Can you work these out from the model? Positions are in its coordinate system, mm. Face numbers are marked on the shaded views. A direction names the side the tool comes from. Round coordinates to 2 decimals unless told otherwise and drop trailing zeros. Write each loop counter-clockwise with the first axis right and the second up, starting at its lowest first coordinate (ties: lowest second). Pieces come first, ordered by that corner, then holes. Notation, with made-up numbers: M 42.25,-25.5 L 68.25,-25.5 A21 cw 68.25,-14.5 Z; hole C 86.25,-36 d8. An arc over 180 degrees is marked long. Answer in a Markdown table with one row per item. Add a question column.
(1) Suppose I cut it at D-D, the plane x = -4. Write out the boundary of the cut face in (y, z), then the cut area to 3 significant figures.
(2) If I drill on probe 1 along Y at (x, z) = (19, -2.2); probe 2 along X at (y, z) = (-20.5, -8.25); probe 3 along Y at (x, z) = (33, -4.5), over which ranges is the centre line in solid material (lowest first)?
(3) Suppose I cut it at B-B, the plane y = -16.5. Write out the boundary of the cut face in (x, z).
(4) Suppose I cut it at C-C, the plane z = -5.75. Write out the boundary of the cut face in (x, y), then the cut area to 3 significant figures.
(5) Suppose I cut it at A-A, the plane x = -30. Write out the boundary of the cut face in (y, z).
(6) For the marked faces 1 and 2, which set-ups out of +Z, -Z, +X, -X, +Y, -Y let a thin tool reach every point of the face, with its end or its side?
(7) I'm going to push flat-ended pins straight in: pin 1 (5 mm diameter, centred on x = -18.5, z = -3, fed in from +Y); pin 2 (2 mm diameter, centred on x = 19, y = 25, fed in from -Z); pin 3 (2.5 mm diameter, centred on x = -39, y = -24.5, fed in from -Z). Where does each tip first touch, or does it pass through?
(8) If we mould it in two halves opening along X, with no side actions, what happens to the marked faces 3, 4, 5 and 6? For each: released by +X, released by -X, zero draft, split by the parting line, or undercut.
Autodesk Inventor part; units mm, degrees
ref_plane "YZ Plane" through (0, 0, 0) normal (1, 0, 0) x (0, 1, 0)
ref_plane "XZ Plane" through (0, 0, 0) normal (0, 1, 0) x (-1, 0, 0)
ref_plane "XY Plane" through (0, 0, 0) normal (0, 0, 1) x (1, 0, 0)
ref_plane "Work Plane1" through (0, 0, 0) normal (0, 0, 1) x (1, 0, 0)
sketch "Sketch1" plane through (0, 0, 0) normal (0, 0, 1) x (1, 0, 0)
  line L0 (47, 31) -> (-47, 31)
  line L1 (-47, 31) -> (-47, -31)
  line L2 (-47, -31) -> (47, -31)
  line L3 (47, -31) -> (47, 31)
  line L4 (47, 31) -> (-47, -31) construction
  line L5 (-47, 31) -> (47, -31) construction
  point P0 (0, 0)
  dimension "d0" = 94
  dimension "d1" = 62
extrude "Extrusion1" add sketch "Sketch1" along normal blind 2
sketch "Sketch2" plane through (0, 0, 0) normal (0, 0, -1) x (-1, 0, 0)
  circle A0 centre (39, 24.5) radius 3
  circle A1 centre (39, 24.5) radius 1.35
  circle A2 centre (39, -24.5) radius 3
  circle A3 centre (39, -24.5) radius 1.35
  circle A4 centre (-19, -24.5) radius 3
  circle A5 centre (-19, -24.5) radius 1.35
  circle A6 centre (-19, 24.5) radius 3
  circle A7 centre (-19, 24.5) radius 1.35
  point P0 (0, 0)
extrude "Extrusion2" add sketch "Sketch2" along normal blind 3
sketch "Sketch3" plane through (0, 0, 0) normal (0, 0, -1) x (-1, 0, 0)
  circle A0 centre (-19, -24.5) radius 3
  circle A1 centre (39, -24.5) radius 3
  circle A2 centre (-19, 24.5) radius 3
  circle A3 centre (39, 24.5) radius 3
  line L0 (47, 31) -> (47, -31)
  line L1 (-47, 31) -> (47, 31)
  line L2 (-47, -31) -> (-47, 31)
  line L3 (47, -31) -> (-47, -31)
  line L4 (45, -29) -> (45, 29)
  line L5 (45, 29) -> (-45, 29)
  line L6 (-45, 29) -> (-45, -29)
  line L7 (-45, -29) -> (45, -29)
  point P0 (0, 0)
  dimension "d6" = 2
extrude "Extrusion3" add sketch "Sketch3" along normal blind 15 contours L0 L3 L2 L1
sketch "Sketch4" plane through (-45, 29, 0) normal (0, -1, 0) x (1, 0, 0)
  point P0 (45, 0)
sketch "Sketch5" plane through (-45, 29, 0) normal (0, -1, 0) x (1, 0, 0)
  line L0 (0, 0) -> (90, 0)
  line L1 (7, 0) -> (37, 0)
  line L2 (37, 0) -> (37, -11)
  line L3 (37, -11) -> (7, -11)
  line L4 (7, -11) -> (7, 0)
  line L5 (0, 0) -> (0, -15)
  line L6 (90, -15) -> (0, -15)
  point P0 (45, 0)
  dimension "d9" = 30
  dimension "d10" = 7
  dimension "d11" = 4
extrude "Extrusion4" cut sketch "Sketch5" against normal blind 15
properties part number "rpi4_case"
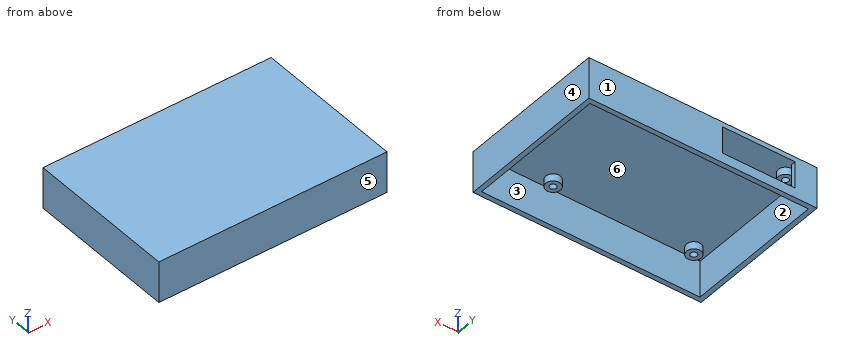
Calculated:
| question | item | result |
|---|---|---|
| 1 | outline | M -31,-15 L -29,-15 L -29,0 L 29,0 L 29,-15 L 31,-15 L 31,2 L -31,2 Z |
| 1 | area | 184 mm² |
| 2 | probe 1 | -31 to -29, -27.5 to -25.85, -23.15 to -21.5, 21.5 to 23.15, 25.85 to 27.5, 29 to 31 |
| 2 | probe 2 | -47 to -45, 45 to 47 |
| 2 | probe 3 | -31 to -29, 29 to 31 |
| 3 | outline | M -47,-15 L -45,-15 L -45,0 L 45,0 L 45,-15 L 47,-15 L 47,2 L -47,2 Z |
| 4 | outline | M -47,-31 L 47,-31 L 47,31 L -8,31 L -8,29 L 45,29 L 45,-29 L -45,-29 L -45,29 L -38,29 L -38,31 L -47,31 Z |
| 4 | area | 548 mm² |
| 5 | outline | M -31,-15 L -29,-15 L -29,0 L 31,0 L 31,2 L -31,2 Z; M 29,-15 L 31,-15 L 31,-11 L 29,-11 Z |
| 6 | face 1 | +Z, -Z, +X, -X, +Y |
| 6 | face 2 | -Z |
| 7 | pin 1 | y = -29 |
| 7 | pin 2 | z = -3 |
| 7 | pin 3 | z = 0 |
| 8 | face 3 | undercut |
| 8 | face 4 | released by +X |
| 8 | face 5 | zero draft |
| 8 | face 6 | undercut |
